from build123d import *

# Parameters (mm, degrees)
CROQUIS1_W              = 118.35
CROQUIS1_H              = 10
SALIENTE_EXTRUIR1_DEPTH = 10
CROQUIS2_W              = 20
CROQUIS2_H              = 5
CORTAR_EXTRUIR1_DEPTH   = 11
CORTAR_EXTRUIR2_DEPTH   = 11
REDONDEO1_R             = 2


with BuildPart() as part:
    # Croquis1 → Saliente-Extruir1 (new body)
    with BuildSketch(Plane.XY):
        Rectangle(CROQUIS1_W, CROQUIS1_H)
    extrude(amount=SALIENTE_EXTRUIR1_DEPTH)

    # Croquis2 → Cortar-Extruir1 (cut, through all)
    with BuildSketch(Plane.XY.offset(10)):
        with Locations((-59.175, 0)):
            Rectangle(CROQUIS2_W, CROQUIS2_H)
    extrude(amount=-CORTAR_EXTRUIR1_DEPTH, mode=Mode.SUBTRACT)

    # Croquis3 → Cortar-Extruir2 (cut, through all)
    with BuildSketch(Plane(origin=(0, 5, 0), x_dir=(1, 0, 0), z_dir=(0, 1, 0))):
        Polygon((59.175, -7), (-30.825, 0), (59.175, 0), align=None)
    extrude(amount=-CORTAR_EXTRUIR2_DEPTH, mode=Mode.SUBTRACT)

    # Redondeo1
    redondeo1_edges = [part.edges().sort_by_distance(p)[0] for p in [
        (-49.175, -2.5, 5),
        (-49.175, 2.5, 5),
    ]]
    fillet(redondeo1_edges, radius=REDONDEO1_R)


solid = part.part
Can you work these out from the model? Positions are in its coordinate system, mm. A direction names the side the tool comes from. Give positions to 0.01 mm unless a question says otherwise; leave off trailing zeros. Order: outer loops, then holes, each group sorted by start corner. A loop starts at its lowest first (then second) coordinate and runs counter-clockwise, first axis right, second up. Notation, with made-up numbers: M 14.25,51 L 19.25,51 A21 ccw 19.25,70 Z; hole C 28.5,59 d7. An arc over 180 degrees is marked long. One line per item, written item: value.
Item 1: If we section it at A-A on z = 8.75: Write out the boundary of the cut face in (x, y) (3 decimals).
Verdict:
outline: M -59.175,-5 L 59.175,-5 L 59.175,5 L -59.175,5 L -59.175,2.5 L -51.175,2.5 A2 cw -49.175,0.5 L -49.175,-0.5 A2 cw -51.175,-2.5 L -59.175,-2.5 Z
Item 2: If we section it at C-C on x = 10: Write out the boundary of the cut face in (y, z).
Verdict:
outline: M -5,3.18 L 5,3.18 L 5,10 L -5,10 Z
Item 3: If we section it at D-D on z = 3: Write out the boundary of the cut face in (x, y) (3 decimals).
Verdict:
outline: M -59.175,-5 L 7.746,-5 L 7.746,5 L -59.175,5 L -59.175,2.5 L -51.175,2.5 A2 cw -49.175,0.5 L -49.175,-0.5 A2 cw -51.175,-2.5 L -59.175,-2.5 Z
Item 4: Please list where these lines run through material, in increasing order: line 1 (Z direction, x = 45.5, y = -0.5); line 2 (Z direction, x = 51, y = 2.5); line 3 (X direction, y = -1.25, z = 7.25) (3 decimals).
Verdict:
line 1: 5.94 to 10
line 2: 6.36 to 10
line 3: -49.321 to 59.175
Item 5: For pin 1 (6 mm diameter, centred on x = 10, y = -3.5, fed in from -Z), with a flat end and sliding along its axis, tell me the tip position at first contact or that it passes through.
Verdict:
pin 1: z = 2.94
Item 6: For faces 4 (the face through (-55, 2.5, 5)), 5 (the face through (14.8, 0.07, 3.55)), which set-ups out of +Z, -Z, +X, -X, +Y, -Y let a thin tool reach every point of the face, with its end or its side?
Verdict:
face 4: +Z, -Z, -X
face 5: -Z, +X, +Y, -Y
Item 7: If we section it at B-B on y = -4: Write out the boundary of the cut face in (x, z) (3 decimals), and give its area (4 significant figures).
Verdict:
outline: M -59.175,0 L -30.825,0 L 59.175,7 L 59.175,10 L -59.175,10 Z
area: 868.5 mm2
Item 8: If we mould it in two halves opening along Y, with no side actions, what happens to faces 1 (the face through (-59.175, 4, 5)), 2 (the face through (-49.776, -1.93, 4.93)), 3 (the face through (-14, 5, 6))? For each: pulls with the +Y half, pulls with the -Y half, needs draft (parallel to the pull), parting line crosses it, or undercut.
Verdict:
face 1: needs draft
face 2: undercut
face 3: pulls with the +Y half
